The model under review builds one solid part; all positions refer to its coordinate system, in mm. Face numbers are marked on the shaded views. A direction names the side the tool comes from. Give positions to 0.01 mm unless a question says otherwise; leave off trailing zeros. Order: outer loops, then holes, each group sorted by start corner. A loop starts at its lowest first (then second) coordinate and runs counter-clockwise, first axis right, second up.
```python
from build123d import *

# Parameters (mm, degrees)
F1_DEPTH = 5
F3_DEPTH = 4.5
F5_DEPTH = 3
F6_R     = 1.5
F7_DEPTH = 8.001


with BuildPart() as f1:
    # F0 (on Top) → F1 (new body)
    with BuildSketch(Plane.XY):
        with BuildLine():
            Line((-3, 0), (0, 3))
            Line((0, 3), (0, 19))
            ThreePointArc((0, 19), (-12.510187, 12.510187), (-19, 0))
            Line((-19, 0), (-3, 0))
        make_face()
    extrude(amount=F1_DEPTH)

    # F2 (on face) → F3 (cut)
    with BuildSketch(Plane.XY.offset(5)):
        Polygon((-10.899495, 1), (-1, 10.899495), (-4.535534, 14.435029), (-14.435029, 4.535534), align=None)
    extrude(amount=-F3_DEPTH, mode=Mode.SUBTRACT)

    # F4 (on face) → F5 (join)
    with BuildSketch(Plane.XY.offset(5)):
        with BuildLine():
            Line((-3.713925, 6.892677), (-6.895905, 3.710697))
            ThreePointArc((-6.895905, 3.710697), (-6.895098, 1.942122), (-5.126524, 1.944544))
            Line((-5.126524, 1.944544), (-1.944544, 5.126524))
            ThreePointArc((-1.944544, 5.126524), (-1.945351, 6.895099), (-3.713925, 6.892677))
        make_face()
    extrude(amount=F5_DEPTH)

    # F6 (on face) → F7 (cut, through all)
    with BuildSketch(Plane.XY):
        with Locations((-7.778175, 7.778175)):
            Circle(F6_R)
    extrude(amount=F7_DEPTH, mode=Mode.SUBTRACT)


solid = f1.part
```
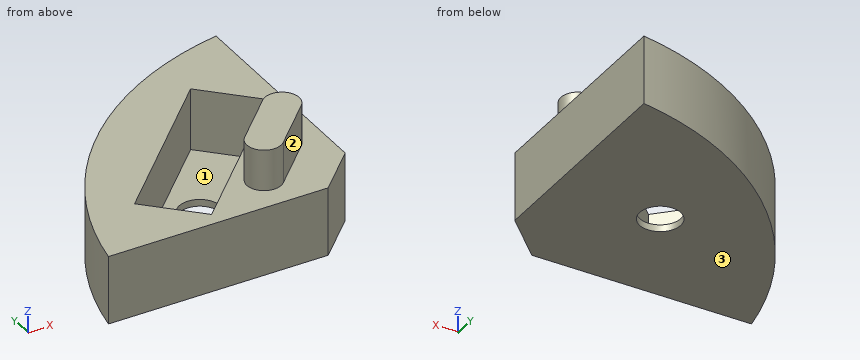
Item 1: For line 1 (Z direction, x = -15.75, y = 4); line 2 (X direction, y = 14.25, z = 3.5); line 3 (X direction, y = 11.5, z = 2.75), list the stretches that pass through material, from the lowest coordinate up.
Values found:
line 1: z = 0 to 5
line 2: x = -10.56 to -4.72, -4.35 to 0
line 3: x = -13.46 to -7.47, -1.6 to 0
Item 2: Clearance check with flat-ended pins moving along their axes: pin 1 Ø4 at (x, y) = (-12, 7) entering from +Z; pin 2 Ø4 at (y, z) = (5.5, 1) entering from -X; pin 3 Ø1 at (x, z) = (-13, 2.5) entering from +Y. State where each tip first meets the part, or that it passes through.
Values found:
pin 1: stops at z = 5
pin 2: stops at x = -18.11
pin 3: stops at y = 12.52
Item 3: Take a section at D-D (x = -2.25). Give the boundary of the cut face in (y, z), and give its area (3 significant figures).
Values found:
outline: (0.75, 0) - (18.49, 0) - (18.49, 5) - (12.15, 5) - (12.15, 0.5) - (9.65, 0.5) - (9.65, 5) - (7.12, 5) - (7.12, 8) - (4.82, 8) - (4.82, 5) - (0.75, 5) - close
area: 84.4 mm2
Item 4: Take a section at A-A (z = 1.75). Give the boundary of the cut face in (x, y).
Values found:
outline: (-19, 0) - (-3, 0) - (0, 3) - (0, 19) arc R23.33 ccw to start; hole (-14.44, 4.54) - (-10.9, 1) - (-1, 10.9) - (-4.54, 14.44) - close
Item 5: Take a section at C-C (y = 11.5). Give the boundary of the cut face in (x, z).
Values found:
outline: (-13.46, 0) - (0, 0) - (0, 5) - (-1.6, 5) - (-1.6, 0.5) - (-7.47, 0.5) - (-7.47, 5) - (-13.46, 5) - close
Item 6: Take a section at B-B (x = -8.25). Give the boundary of the cut face in (y, z).
Values found:
outline: (0, 0) - (6.35, 0) - (6.35, 0.5) - (3.65, 0.5) - (3.65, 5) - (0, 5) - close; (9.2, 0) - (15.88, 0) - (15.88, 5) - (10.72, 5) - (10.72, 0.5) - (9.2, 0.5) - close
Item 7: For the marked faces 1, 2 and 3, list the 3-axis set-ups (+Z, -Z, +X, -X, +Y, -Y) from which the entire face can be reached by the end or side of a thin tool; tool diameter is ignored.
Values found:
face 1: +Z
face 2: +Z, +X, -Y
face 3: -Z, +X, -X, +Y, -Y
